Autodesk Fusion 360 part; units mm, degrees
sketch "Base" plane through (0, 0, 0) normal (0, 0, 1) x (1, 0, 0) in component "Colour Sensor Holder Bottom"
  line L0 (0, 0) -> (46.334, 0)
  line L1 (46.334, 0) -> (46.334, 30)
  line L2 (46.334, 30) -> (0, 30)
  line L3 (0, 30) -> (0, 0)
  dimension "d2" = 46.334
  dimension "d3" = 30
extrude "Extrude1" add sketch "Base" along normal blind 4 in component "Colour Sensor Holder Bottom"
sketch "Side Profile" plane through (0, 0, 0) normal (0, -1, 0) x (1, 0, 0) in component "Colour Sensor Holder Bottom"
  line L0 (0, 0) -> (46.334, 0)
  line L1 (46.334, 0) -> (46.334, 4)
  line L2 (46.334, 4) -> (0, 4)
  line L3 (0, 4) -> (0, 0)
  line L4 (46.334, 4) -> (46.334, 16)
  line L5 (46.334, 16) -> (80.334, 16)
  line L6 (80.334, 16) -> (80.334, 30)
  line L7 (80.334, 30) -> (0, 30)
  line L8 (0, 30) -> (0, 4)
  dimension "d6" = 12
  dimension "d7" = 34
  dimension "d8" = 14
  dimension "d11" = 46.334
  dimension "d52" = 80.334
extrude "Extrude2" add sketch "Side Profile" against normal blind 4.5 contours L2 L4 L5 L6 L7 L8 in component "Colour Sensor Holder Bottom"
extrude "Extrude3" add sketch "Side Profile" against normal blind 4.5 from surface at -25.5 contours L2 L4 L5 L6 L7 L8 in component "Colour Sensor Holder Bottom"
sketch "Front End" plane through (0, 0, 0) normal (0, -1, 0) x (1, 0, 0) in component "Colour Sensor Holder Bottom"
  line L0 (0, 0) -> (46.334, 0)
  line L1 (46.334, 0) -> (46.334, 16)
  line L2 (46.334, 16) -> (80.334, 16)
  line L3 (80.334, 16) -> (80.334, 30)
  line L4 (80.334, 30) -> (0, 30)
  line L5 (0, 30) -> (0, 0)
  line L6 (80.334, 30) -> (76.034, 30)
  line L7 (76.034, 30) -> (76.034, 16)
  line L8 (76.034, 16) -> (80.334, 16)
  line L9 (80.334, 16) -> (80.334, 30)
  dimension "d17" = 4.3
extrude "Extrude4" add sketch "Front End" against normal blind 30 contours L2 L3 L4 L6 L7 L8 L9 in component "Colour Sensor Holder Bottom"
sketch "Middle End" plane through (0, 0, 0) normal (0, -1, 0) x (1, 0, 0) in component "Colour Sensor Holder Bottom"
  line L0 (80.334, 30) -> (0, 30)
  line L1 (0, 30) -> (0, 0)
  line L2 (0, 0) -> (46.334, 0)
  line L3 (46.334, 0) -> (46.334, 16)
  line L4 (46.334, 16) -> (80.334, 16)
  line L5 (80.334, 16) -> (80.334, 30)
  line L6 (46.334, 23) -> (40.334, 23)
  line L7 (40.334, 23) -> (40.334, 0)
  line L8 (40.334, 0) -> (46.334, 0)
  line L9 (46.334, 0) -> (46.334, 23)
  dimension "d20" = 7
  dimension "d21" = 6
extrude "Extrude5" add sketch "Middle End" against normal blind 30 contours L2 L3 L6 L7 L8 L9 in component "Colour Sensor Holder Bottom"
sketch "Lip" plane through (76.034, 0, 0) normal (-1, 0, 0) x (0, -1, 0) in component "Colour Sensor Holder Bottom"
  line L0 (-25.5, 30) -> (-25.5, 16)
  line L1 (-25.5, 16) -> (-4.5, 16)
  line L2 (-4.5, 16) -> (-4.5, 30)
  line L3 (-4.5, 30) -> (-25.5, 30)
  line L4 (-18, 25) -> (-12, 25)
  line L5 (-12, 25) -> (-12, 21)
  line L6 (-12, 21) -> (-18, 21)
  line L7 (-18, 21) -> (-18, 25)
  dimension "d24" = 5
  dimension "d25" = 6
  dimension "d26" = 4
  dimension "d27" = 7.5
extrude "Extrude6" add sketch "Lip" along normal blind 4 contours L4 L5 L6 L7 in component "Colour Sensor Holder Bottom"
sketch "Magnet Holders" plane through (0, 0, 30) normal (0, 0, 1) x (-1, 0, 0) in component "Colour Sensor Holder Bottom"
  line L0 (-80.334, -30) -> (0, -30)
  line L1 (0, -30) -> (0, -25.5)
  line L2 (0, -25.5) -> (-76.034, -25.5)
  line L3 (-76.034, -25.5) -> (-76.034, -4.5)
  line L4 (-76.034, -4.5) -> (0, -4.5)
  line L5 (0, -4.5) -> (0, 0)
  line L6 (0, 0) -> (-80.334, 0)
  line L7 (-80.334, 0) -> (-80.334, -30)
  circle A0 centre (-68.334, -30) radius 5
  circle A1 centre (-38.334, -30) radius 5
  circle A2 centre (-38.334, 0) radius 5
  circle A3 centre (-68.334, 0) radius 5
  circle A4 centre (-38.334, 0) radius 2.75
  circle A5 centre (-68.334, 0) radius 2.75
  circle A6 centre (-38.334, -30) radius 2.75
  circle A7 centre (-68.334, -30) radius 2.75
  dimension "d33" = 10
  dimension "d34" = 10
  dimension "d35" = 10
  dimension "d36" = 10
  dimension "d37" = 12
  dimension "d38" = 12
  dimension "d43" = 5.5
  dimension "d44" = 5.5
  dimension "d45" = 5.5
  dimension "d46" = 5.5
  dimension "d50" = 42
  dimension "d51" = 42
extrude "Extrude8" add sketch "Magnet Holders" against normal blind 4 contours L0 A7 | L0 A0 A7 | L0 A1 A6 | L0 A6 | L6 A3 A5 | L6 A5 | L6 A2 A4 | L6 A4 picked at (-68.2655, -30.9141) picked at (-37.4674, -30.6679) picked at (-68.2655, 0.9141) picked at (-39.0365, 1.0303) in component "Colour Sensor Holder Bottom"
extrude "Extrude9" cut sketch "Magnet Holders" against normal blind 1.5 contours L0 A7 | L0 A7 | L0 A6 | L0 A6 | L6 A5 | L6 A5 | L6 A4 | L6 A4 in component "Colour Sensor Holder Bottom"
sketch "Conduit Angle" plane through (0, 0, 30) normal (0, 0, 1) x (-1, 0, 0) in component "Colour Sensor Holder Bottom"
  circle A0 centre (-68.334, 0) radius 2.75
  circle A1 centre (-38.334, -30) radius 2.75
  circle A2 centre (-38.334, 0) radius 2.75
  circle A3 centre (-68.334, -30) radius 2.75
  line L0 (-33.334, -30) -> (0, -30)
  line L1 (0, -30) -> (0, -25.5)
  line L2 (0, -25.5) -> (-76.034, -25.5)
  line L3 (-76.034, -25.5) -> (-76.034, -4.5)
  line L4 (-76.034, -4.5) -> (0, -4.5)
  line L5 (0, -4.5) -> (0, 0)
  line L6 (0, 0) -> (-33.334, 0)
  arc A4 (-33.334, 0) -> (-43.334, 0) centre (-38.334, 0) ccw
  line L7 (-43.334, 0) -> (-63.334, 0)
  arc A5 (-63.334, 0) -> (-73.334, 0) centre (-68.334, 0) ccw
  line L8 (-73.334, 0) -> (-80.334, 0)
  line L9 (-80.334, 0) -> (-80.334, -30)
  line L10 (-80.334, -30) -> (-73.334, -30)
  arc A6 (-73.334, -30) -> (-63.334, -30) centre (-68.334, -30) ccw
  line L11 (-63.334, -30) -> (-43.334, -30)
  arc A7 (-43.334, -30) -> (-33.334, -30) centre (-38.334, -30) ccw
  line L12 (-40.334, -4.5) -> (-40.334, -25.5)
  line L13 (-40.334, -25.5) -> (0, -25.5)
  line L14 (0, -25.5) -> (0, -4.5)
  line L15 (0, -4.5) -> (-40.334, -4.5)
  line L16 (0, -30) -> (-19.932, 0)
  dimension "d53" = 33.6
extrude "Extrude10" cut sketch "Conduit Angle" against normal blind 30 contours L1 L2 L13 L16 | L2 L4 L13 L14 L15 L16 | L4 L5 L6 L15 L16 in component "Colour Sensor Holder Bottom"
sketch "Conduit Height" plane through (13.8279, 9.1873, 0) normal (-0.8329, -0.5534, 0) x (0.5534, -0.8329, 0) in component "Colour Sensor Holder Bottom"
  line L0 (-19.585, 4) -> (-19.585, 30)
  line L1 (-19.585, 30) -> (-24.9876, 30)
  line L2 (-24.9876, 30) -> (-24.9876, 0)
  line L3 (-24.9876, 0) -> (11.0302, 0)
  line L4 (11.0302, 0) -> (11.0302, 30)
  line L5 (11.0302, 30) -> (5.6275, 30)
  line L6 (5.6275, 30) -> (5.6275, 4)
  line L7 (5.6275, 4) -> (-19.585, 4)
  line L8 (-24.9876, 0) -> (11.0302, 0)
  line L9 (11.0302, 0) -> (11.0302, 16)
  line L10 (11.0302, 16) -> (-24.9876, 16)
  line L11 (-24.9876, 16) -> (-24.9876, 0)
  point P0 (5.6275, 16)
  point P1 (-19.585, 16)
  dimension "d56" = 16
sketch "Colour Sensor Cover Shape" plane through (0, 0, 30) normal (0, 0, 1) x (-1, 0, 0) in component "Colour Sensor Holder Bottom"
  line L0 (0, -30) -> (-2.9898, -25.5)
  line L1 (-2.9898, -25.5) -> (-76.034, -25.5)
  line L2 (-76.034, -25.5) -> (-76.034, -4.5)
  line L3 (-76.034, -4.5) -> (-16.9422, -4.5)
  line L4 (-16.9422, -4.5) -> (-19.932, 0)
  line L5 (-19.932, 0) -> (-33.334, 0)
  arc A0 (-33.334, 0) -> (-43.334, 0) centre (-38.334, 0) ccw
  line L6 (-43.334, 0) -> (-63.334, 0)
  arc A1 (-63.334, 0) -> (-73.334, 0) centre (-68.334, 0) ccw
  line L7 (-73.334, 0) -> (-80.334, 0)
  line L8 (-80.334, 0) -> (-80.334, -30)
  line L9 (-80.334, -30) -> (-73.334, -30)
  arc A2 (-73.334, -30) -> (-63.334, -30) centre (-68.334, -30) ccw
  line L10 (-63.334, -30) -> (-43.334, -30)
  arc A3 (-43.334, -30) -> (-33.334, -30) centre (-38.334, -30) ccw
  line L11 (-33.334, -30) -> (0, -30)
  circle A4 centre (-68.334, 0) radius 2.75
  circle A5 centre (-38.334, -30) radius 2.75
  circle A6 centre (-38.334, 0) radius 2.75
  circle A7 centre (-68.334, -30) radius 2.75
  line L12 (-33.334, -30) -> (-33.334, 0)
  point P0 (-33.334, -25.5)
  point P1 (-33.334, -4.5)
sketch "Right Loft Outside Shape" plane through (0, 0, 0) normal (0, -1, 0) x (1, 0, 0) in component "Colour Sensor Holder Bottom"
  line L0 (19.932, 30) -> (19.932, 0)
  line L1 (19.932, 0) -> (46.334, 0)
  line L2 (46.334, 0) -> (46.334, 16)
  line L3 (46.334, 16) -> (80.334, 16)
  line L4 (80.334, 16) -> (80.334, 30)
  line L5 (80.334, 30) -> (73.334, 30)
  line L6 (73.334, 30) -> (73.334, 26)
  line L7 (73.334, 26) -> (63.334, 26)
  line L8 (63.334, 26) -> (63.334, 30)
  line L9 (63.334, 30) -> (43.334, 30)
  line L10 (43.334, 30) -> (43.334, 26)
  line L11 (43.334, 26) -> (33.334, 26)
  line L12 (33.334, 26) -> (33.334, 30)
  line L13 (33.334, 30) -> (19.932, 30)
  line L14 (33.334, 30) -> (19.932, 16)
  point P0 (33.334, 30)
  point P1 (19.932, 16)
sketch "Right Loft Inside Shape" plane through (0, 4.5, 0) normal (0, 1, 0) x (-1, 0, 0) in component "Colour Sensor Holder Bottom"
  line L0 (-16.9422, 4) -> (-16.9422, 30)
  line L1 (-16.9422, 30) -> (-76.034, 30)
  line L2 (-76.034, 30) -> (-76.034, 16)
  line L3 (-76.034, 16) -> (-46.334, 16)
  line L4 (-46.334, 16) -> (-46.334, 23)
  line L5 (-46.334, 23) -> (-40.334, 23)
  line L6 (-40.334, 23) -> (-40.334, 4)
  line L7 (-40.334, 4) -> (-16.9422, 4)
  line L8 (-33.334, 30) -> (-16.9422, 16)
  point P0 (-33.334, 30)
  point P1 (-16.9422, 16)
sketch "Left Loft Inside Shape" plane through (0, 25.5, 0) normal (0, -1, 0) x (1, 0, 0) in component "Colour Sensor Holder Bottom"
  line L0 (2.9898, 30) -> (2.9898, 4)
  line L1 (2.9898, 4) -> (40.334, 4)
  line L2 (40.334, 4) -> (40.334, 23)
  line L3 (40.334, 23) -> (46.334, 23)
  line L4 (46.334, 23) -> (46.334, 16)
  line L5 (46.334, 16) -> (76.034, 16)
  line L6 (76.034, 16) -> (76.034, 30)
  line L7 (76.034, 30) -> (2.9898, 30)
  line L8 (33.334, 30) -> (2.9898, 16)
  point P0 (33.334, 30)
  point P1 (2.9898, 16)
sketch "Left Loft Outside Shape" plane through (0, 30, 0) normal (0, 1, 0) x (-1, 0, 0) in component "Colour Sensor Holder Bottom"
  line L0 (-33.334, 30) -> (-33.334, 26)
  line L1 (-33.334, 26) -> (-43.334, 26)
  line L2 (-43.334, 26) -> (-43.334, 30)
  line L3 (-43.334, 30) -> (-63.334, 30)
  line L4 (-63.334, 30) -> (-63.334, 26)
  line L5 (-63.334, 26) -> (-73.334, 26)
  line L6 (-73.334, 26) -> (-73.334, 30)
  line L7 (-73.334, 30) -> (-80.334, 30)
  line L8 (-80.334, 30) -> (-80.334, 16)
  line L9 (-80.334, 16) -> (-46.334, 16)
  line L10 (-46.334, 16) -> (-46.334, 0)
  line L11 (-46.334, 0) -> (0, 0)
  line L12 (0, 0) -> (0, 30)
  line L13 (0, 30) -> (-33.334, 30)
  line L14 (-33.334, 30) -> (0, 16)
  point P0 (-33.334, 30)
  point P1 (0, 16)
loft "Loft1" cut profiles "Right Loft Outside Shape", "Right Loft Inside Shape" section 1 contours L0 L13 L14 section 2 contours L0 L1 L8 in component "Colour Sensor Holder Bottom"
loft "Loft2" cut profiles "Left Loft Inside Shape", "Left Loft Outside Shape" section 1 contours L0 L7 L8 section 2 contours L12 L13 L14 in component "Colour Sensor Holder Bottom"
chamfer "Chamfer2" distance 4 distance2 2 1 edges at (9.966, 15, 4) measured on face at (20.0887, 18.5, 4) in component "Colour Sensor Holder Bottom"
sketch "Top and Middle Segments" plane through (0, 0, 0) normal (0, -1, 0) x (1, 0, 0)
  line L0 (33.334, 30) -> (19.932, 16)
  line L1 (19.932, 16) -> (19.932, 0)
  line L2 (19.932, 0) -> (46.334, 0)
  line L3 (46.334, 0) -> (46.334, 16)
  line L4 (46.334, 16) -> (80.334, 16)
  line L5 (80.334, 16) -> (80.334, 30)
  line L6 (80.334, 30) -> (73.334, 30)
  line L7 (73.334, 30) -> (73.334, 26)
  line L8 (73.334, 26) -> (63.334, 26)
  line L9 (63.334, 26) -> (63.334, 30)
  line L10 (63.334, 30) -> (43.334, 30)
  line L11 (43.334, 30) -> (43.334, 26)
  line L12 (43.334, 26) -> (33.334, 26)
  line L13 (33.334, 26) -> (33.334, 30)
  line L14 (16.9422, 16) -> (16.9422, 2)
  line L15 (16.9422, 2) -> (2.9898, 2)
  line L16 (2.9898, 2) -> (2.9898, 16)
  line L17 (2.9898, 16) -> (0, 16)
  line L18 (0, 16) -> (0, 0)
  line L19 (0, 0) -> (19.932, 0)
  line L20 (19.932, 0) -> (19.932, 16)
  line L21 (19.932, 16) -> (16.9422, 16)
  line L22 (0, 16) -> (80.334, 16)
  line L23 (80.334, 16) -> (80.334, 30)
  line L24 (80.334, 30) -> (0, 30)
  line L25 (0, 30) -> (0, 16)
extrude "Extrude11" cut sketch "Top and Middle Segments" along normal blind -35 and the other way blind -5 contours L0 L4 L5 L6 L7 L8 L9 L10 L11 L12 L13 L22 L23 L24 | L11 L12 L13 L24 | L0 L17 L21 L22 L24 L25 | L7 L8 L9 L24 in component "Colour Sensor Holder Bottom"
component "Colour Sensor Holder Bottom" placed x (1, 0, 0) y (0, 1, 0) z (0, 0, 1) at (0, 0, 0)
equation "base_plate_thickness = 4 mm"
equation "d4 = base_plate_thickness"
equation "d37 = 7 mm + 5 mm"
equation "d38 = 7 mm + 5 mm"
CAD build for the part. Positions are in the model's coordinates, mm. A direction names the side the tool comes from. Give positions to 0.01 mm unless a question says otherwise; leave off trailing zeros. Loops run counter-clockwise (first coordinate to the right, second up) from the corner with the lowest first, then second, coordinate; pieces in that order, holes last. Notation, with made-up numbers: M -13,67 L 9,67 A26 cw 9,89 Z; hole C -13,-33.5 d1. An arc over 180 degrees is marked long. One line per question, with ' | ' between items. Start each with the question number.
1. Saw through at B-B on y = 8.5. Give the cut face in (x, z).
2. 3-axis set-ups, long thin cutter, end or side, ignore diameter. For faces 4 (the face through (21, 25.5, 9)), 5 (the face through (46.334, 15, 8)): which of +Z, -Z, +X, -X, +Y, -Y reach the whole face in a straight line?
3. Saw through at A-A on x = 25.5. Give the cut face in (y, z).
4. Saw through at C-C on z = 10.5. Give the cut face in (x, y), plus the area to 3 significant figures.
5. Probe L1, parallel to Y at x = 32, z = 13.25; L2, parallel to Z at x = 10, y = 24.5; L3, parallel to X at y = 9.5, z = 10. List the from-to ranges inside material, lowest first. Write a range as from..to.
6. Two-plate mould, pull along Y, no slides. Class faces 1 (the face through (9.9, 15.1, 1.5)), 2 (the face through (27, 15, 4)), 3 (the face through (23, 30, 8)): pulls with the +Y half, pulls with the -Y half, needs draft (parallel to the pull), parting line crosses it, or undercut.
7. Flat gauge pins, fed straight in: pin 1 (3 mm diameter, centred on x = 7.5, z = 8.5, fed in from -Y); pin 2 (8 mm diameter, centred on x = 10, y = 7.5, fed in from +Z); pin 3 (4 mm diameter, centred on x = 16.5, z = 12.5, fed in from -Y); pin 4 (2 mm diameter, centred on x = 15.5, y = 21.5, fed in from +Z). Where does each tip first touch, or does it go through?
8. Saw through at D-D on z = 1.5. Give the cut face in (x, y).
Result sheet:
1) outline: M 14.28,0 L 46.33,0 L 46.33,16 L 40.33,16 L 40.33,4 L 19.09,4 L 14.28,2 Z
2) face 4: +Z, -X | face 5: +Z, -Z, +X, +Y, -Y
3) outline: M 0,0 L 30,0 L 30,16 L 25.5,16 L 25.5,4 L 4.5,4 L 4.5,16 L 0,16 Z
4) outline: M 0,30 L 2.99,25.5 L 40.33,25.5 L 40.33,4.5 L 16.94,4.5 L 19.93,0 L 46.33,0 L 46.33,30 Z | area: 453 mm^2
5) L1: y = 0..4.5, 25.5..30 | L2: z = 0..4 | L3: x = 40.33..46.33
6) face 1: pulls with the -Y half | face 2: undercut | face 3: pulls with the +Y half
7) pin 1: stops at y = 25.5 | pin 2: passes through | pin 3: stops at y = 2.16 | pin 4: stops at z = 4
8) outline: M 0,30 L 19.93,0 L 46.33,0 L 46.33,30 Z
